The model under review builds one solid part; all positions refer to its coordinate system, in mm. A direction names the side the tool comes from. Round coordinates to 2 decimals unless told otherwise and drop trailing zeros. Loops run counter-clockwise (first coordinate to the right, second up) from the corner with the lowest first, then second, coordinate; pieces in that order, holes last. Notation, with made-up numbers: (10, -31.5) -> (49, -31.5) arc R16 ccw to (49, -6.5) -> close; hole circle Ø9 at (55.25, -16). An arc over 180 degrees is marked (long way). Use a Markdown table: item, result. Add a question column.
1) Mouldability with a two-part tool opening along Z and no side actions: class faces 5 (the cylindrical face through (14.454, -4.529, 8.685)), 6 (the flat face through (-6.3, -0.1, 12)), 7 (the cylindrical face through (-0.199, 9.048, 5.916)) as released by +Z, released by -Z, zero draft, split by the parting line, or undercut.
2) Wall thickness on probe 1 along X at (y, z) = (-4.2, 6); probe 2 along Z at (x, y) = (-15.05, -5); probe 3 along X at (y, z) = (-0.75, 11): over which ranges is each line inside the solid? List them lowest first.
3) Consider section D-D on z = 11.25. Give the boundary of the cut face in (x, y), plus the area to 3 significant figures.
4) Consider section C-C on y = 5.25. Give the boundary of the cut face in (x, z).
5) Consider section A-A on x = -15.05. Give the boundary of the cut face in (y, z), plus the area to 3 significant figures.
6) Insertion check: pin 1 (6 mm diameter, centred on x = 14.5, z = 5, fed in from +Y); pin 2 (1.5 mm diameter, centred on y = 2, z = 6, fed in from -X); pin 3 (5 mm diameter, centred on x = 2, z = 4, fed in from +Y); pin 4 (0.9 mm diameter, centred on y = -1, z = 3.5, fed in from +X). Each pin has a flat end and moves straight along its axis. Give the tip position at first contact, or say it passes through.
7) Consider section B-B on z = 6. Give the boundary of the cut face in (x, y), plus the area to 3 significant figures.
8) For faces 1 (the flat face through (-6.3, -0.1, 0)), 2 (the flat face through (18, -3.05, 6)), 3 (the cylindrical face through (6.335, -5.749, 6.084)), 4 (the flat face through (-18, -3.05, 6)), list the 3-axis set-ups (+Z, -Z, +X, -X, +Y, -Y) from which the entire face can be reached by the end or side of a thin tool; tool diameter is ignored.
Autodesk Inventor part; units mm, degrees
ref_plane "YZ Plane" through (0, 0, 0) normal (1, 0, 0) x (0, 1, 0)
ref_plane "XZ Plane" through (0, 0, 0) normal (0, 1, 0) x (-1, 0, 0)
ref_plane "XY Plane" through (0, 0, 0) normal (0, 0, 1) x (1, 0, 0)
sketch "Sketch1" plane through (0, 0, 0) normal (0, 0, 1) x (1, 0, 0)
  circle A0 centre (0, 0) radius 6.05
  circle A1 centre (0, 0) radius 9.05
  line L0 (-21.05, -6.05) -> (21.05, -6.05)
  line L1 (-9.05, 0) -> (-9.05, -6.05)
  line L2 (-6.05, 0) -> (-6.05, -6.05)
  line L3 (6.05, 0) -> (6.05, -6.05)
  line L4 (9.05, 0) -> (9.05, -6.05)
  line L5 (21.05, -6.05) -> (21.05, -3.05)
  line L6 (21.05, -3.05) -> (9.05, -3.05)
  line L7 (-21.05, -6.05) -> (-21.05, -3.05)
  line L8 (-21.05, -3.05) -> (-9.05, -3.05)
  dimension "d0" = 12.1
  dimension "d1" = 3
  dimension "d2" = 12
  dimension "d3" = 3
  dimension "d4" = 3
  dimension "d5" = 12
extrude "Extrusion1" add sketch "Sketch1" along normal blind 12 contours A0 L2 L0 A1 L3 | A1 L4 L0 | L0 L1 A1 | L4 L6 L5 L0 | L0 L7 L8 L1
fillet "Fillet1" radius 1 2 edges at (6.05, -6.05, 6) (-6.05, -6.05, 6)
sketch "Sketch2" plane through (9.05, -3.05, 0) normal (0, 1, 0) x (1, 0, 0)
  line L0 (12, 0) -> (12, -12)
  line L1 (12, -6) -> (0, -6)
  line L2 (0, 0) -> (0, -12)
  line L3 (-18.1, -12) -> (0, -12)
  line L4 (-9.05, -12) -> (-9.05, -16.2316)
  circle A0 centre (6, -6) radius 2.75
  circle A1 centre (-24.1, -6) radius 2.75
  point P0 (-9.05, 0)
  dimension "d9" = 5.5
extrude "Extrusion2" cut sketch "Sketch2" against normal blind 12
equation "\"d4\" = d3"
equation "\"d5\" = d2"
properties part number "Pipe Clamp_3DPrint"
Result set:
| question | item | result |
|---|---|---|
| 1 | face 5 | undercut |
| 1 | face 6 | released by +Z |
| 1 | face 7 | zero draft |
| 2 | probe 1 | -21.05 to -17.8, -12.3 to -6.05, 6.05 to 12.3, 17.8 to 21.05 |
| 2 | probe 2 | 0 to 3.25, 8.75 to 12 |
| 2 | probe 3 | -9.05 to -6.05, 6.05 to 9.05 |
| 3 | outline | (-21.05, -6.05) -> (-7.05, -6.05) arc R1 ccw to (-6.05, -5.05) -> (-6.05, 0) arc R6.05 cw to (6.05, 0) -> (6.05, -5.05) arc R1 ccw to (7.05, -6.05) -> (21.05, -6.05) -> (21.05, -3.05) -> (9.05, -3.05) -> (9.05, 0) arc R9.05 ccw to (-9.05, 0) -> (-9.05, -3.05) -> (-21.05, -3.05) -> close |
| 3 | area | 179 mm2 |
| 4 | outline | (-7.37, 0) -> (-3.01, 0) -> (-3.01, 12) -> (-7.37, 12) -> close; (3.01, 0) -> (7.37, 0) -> (7.37, 12) -> (3.01, 12) -> close |
| 5 | outline | (-6.05, 0) -> (-3.05, 0) -> (-3.05, 3.25) -> (-6.05, 3.25) -> close; (-6.05, 8.75) -> (-3.05, 8.75) -> (-3.05, 12) -> (-6.05, 12) -> close |
| 5 | area | 19.5 mm2 |
| 6 | pin 1 | y = -3.05 |
| 6 | pin 2 | x = -8.96 |
| 6 | pin 3 | y = 9.05 |
| 6 | pin 4 | x = 9.05 |
| 7 | outline | (-21.05, -6.05) -> (-17.8, -6.05) -> (-17.8, -3.05) -> (-21.05, -3.05) -> close; (-12.3, -6.05) -> (-7.05, -6.05) arc R1 ccw to (-6.05, -5.05) -> (-6.05, 0) arc R6.05 cw to (6.05, 0) -> (6.05, -5.05) arc R1 ccw to (7.05, -6.05) -> (12.3, -6.05) -> (12.3, -3.05) -> (9.05, -3.05) -> (9.05, 0) arc R9.05 ccw to (-9.05, 0) -> (-9.05, -3.05) -> (-12.3, -3.05) -> close; (17.8, -6.05) -> (21.05, -6.05) -> (21.05, -3.05) -> (17.8, -3.05) -> close |
| 7 | area | 146 mm2 |
| 8 | face 1 | -Z, +X, -X, +Y, -Y |
| 8 | face 2 | +Z, -Z, +X, +Y |
| 8 | face 3 | +Z, -Z, -Y |
| 8 | face 4 | +Z, -Z, -X, +Y |
